Can you work these out from the model? Positions are in its coordinate system, mm. A direction names the side the tool comes from. Give positions to 0.01 mm unless a question says otherwise; leave off trailing zeros. Loops run counter-clockwise (first coordinate to the right, second up) from the corner with the lowest first, then second, coordinate; pieces in that order, holes last. Notation, with made-up numbers: (37.25, 70.5) -> (64.25, 70.5) arc R8 cw to (64.25, 83.5) -> close; hole circle Ø1 at (25.25, 35). An arc over 180 degrees is marked (long way). Return JSON: item names as keys, results as strings. Group by question number.
Q1. I need wall thicknesses on line 1 along X through (y, z) = (4.25, 10.5); line 2 along Y through (x, z) = (11, 0.75); line 3 along X through (y, z) = (13.5, 1.5) (3 decimals). Which ranges of each line are inside material? Lowest first, please. Write a range as [from, to].
Q2. Will these pins go through, and if not, where does the flat tip stop? pin 1 (0.8 mm diameter, centred on x = 0, z = 5.5, fed in from -Y); pin 2 (1 mm diameter, centred on y = 5, z = 2, fed in from -X); pin 3 (1.5 mm diameter, centred on x = 2.5, z = 5.5, fed in from +Y); pin 4 (1.5 mm diameter, centred on x = -4, y = 3, fed in from +Z).
Q3. Suppose I cut it at B-B, the plane z = 6. Please give me the cut outline in (x, y).
Q4. Suppose I cut it at C-C, the plane z = 1.5. Please give me the cut outline in (x, y).
Q5. Which directions (+Z, -Z, +X, -X, +Y, -Y) give clear straight access to the entire face, cutting with the end or side of a thin tool? Please do faces 1 (the cylindrical face through (3.101, 1.585, 5.916)), 2 (the flat face through (-2.8, 5, 6)), 3 (the cylindrical face through (2.16, 0.69, 5.92)).
Q6. Thinking about a two-plate mould opening in Y: for faces 4 (the flat face through (-1.5, 5, 6)), 5 (the cylindrical face through (2.14, 10.35, 9.34)), 6 (the cylindrical face through (-2.16, 10.35, 9.34)), 7 (the flat face through (10, 0, 6)), which applies, pulls with the +Y half, pulls with the -Y half, needs draft (parallel to the pull), parting line crosses it, or undercut?
Q7. Suppose I cut it at A-A, the plane y = 9.3. Please give me the cut outline in (x, z).
Q8. Suppose I cut it at D-D, the plane y = 7.5. Please give me the cut outline in (x, z).
```python
from build123d import *

# Parameters (mm, degrees)
EXTRUDE_1_DEPTH       = 12
HOLE_WIZARD_7_0_7_1_D = 7


with BuildPart() as part:
    # 草图1 → 拉伸-薄壁1 (new body)
    with BuildSketch(Plane.XY):
        with BuildLine():
            Line((-16.7, 0), (-3.8, 0))
            ThreePointArc((-3.8, 0), (-2.173654403, 0.673654403), (-1.5, 2.3))
            Line((-1.5, 2.3), (-1.5, 13))
            ThreePointArc((-1.5, 13), (-1.207106781, 13.707106781), (-0.5, 14))
            Line((-0.5, 14), (0.5, 14))
            ThreePointArc((0.5, 14), (1.207106781, 13.707106781), (1.5, 13))
            Line((1.5, 13), (1.5, 2.3))
            ThreePointArc((1.5, 2.3), (2.173654403, 0.673654403), (3.8, 0))
            Line((3.8, 0), (16.7, 0))
            Line((16.7, 0), (16.7, 1.3))
            Line((16.7, 1.3), (3.8, 1.3))
            ThreePointArc((3.8, 1.3), (3.092893219, 1.592893219), (2.8, 2.3))
            Line((2.8, 2.3), (2.8, 13))
            ThreePointArc((2.8, 13), (2.126345597, 14.626345597), (0.5, 15.3))
            Line((0.5, 15.3), (-0.5, 15.3))
            ThreePointArc((-0.5, 15.3), (-2.126345597, 14.626345597), (-2.8, 13))
            Line((-2.8, 13), (-2.8, 2.3))
            ThreePointArc((-2.8, 2.3), (-3.092893219, 1.592893219), (-3.8, 1.3))
            Line((-3.8, 1.3), (-16.7, 1.3))
            Line((-16.7, 1.3), (-16.7, 0))
        make_face()
    extrude(amount=EXTRUDE_1_DEPTH)

    # Ø7.0 (7) 直径孔1 (through all)
    with Locations(Plane(origin=(2.8, 0, 0), x_dir=(0, 0, -1), z_dir=(1, 0, 0))):
        with Locations((-6, 9.3)):
            Hole(HOLE_WIZARD_7_0_7_1_D / 2)


solid = part.part
```
Ans:
{
 "1": {"line 1": "x = [-2.8, -1.5], [1.5, 2.8]", "line 2": "y = [0, 1.3]", "line 3": "x = [-2.745, -1.366], [1.366, 2.745]"},
 "2": {"pin 1": "stops at y = 14", "pin 2": "stops at x = -2.8", "pin 3": "stops at y = 14.93", "pin 4": "passes through"},
 "3": {"outline": "(-16.7, 0) -> (-3.8, 0) arc R2.3 ccw to (-1.5, 2.3) -> (-1.5, 5.8) -> (-2.8, 5.8) -> (-2.8, 2.3) arc R1 cw to (-3.8, 1.3) -> (-16.7, 1.3) -> close; (-2.8, 12.8) -> (-1.5, 12.8) -> (-1.5, 13) arc R1 cw to (-0.5, 14) -> (0.5, 14) arc R1 cw to (1.5, 13) -> (1.5, 12.8) -> (2.8, 12.8) -> (2.8, 13) arc R2.3 ccw to (0.5, 15.3) -> (-0.5, 15.3) arc R2.3 ccw to (-2.8, 13) -> close; (1.5, 2.3) arc R2.3 ccw to (3.8, 0) -> (16.7, 0) -> (16.7, 1.3) -> (3.8, 1.3) arc R1 cw to (2.8, 2.3) -> (2.8, 5.8) -> (1.5, 5.8) -> close"},
 "4": {"outline": "(-16.7, 0) -> (-3.8, 0) arc R2.3 ccw to (-1.5, 2.3) -> (-1.5, 13) arc R1 cw to (-0.5, 14) -> (0.5, 14) arc R1 cw to (1.5, 13) -> (1.5, 2.3) arc R2.3 ccw to (3.8, 0) -> (16.7, 0) -> (16.7, 1.3) -> (3.8, 1.3) arc R1 cw to (2.8, 2.3) -> (2.8, 13) arc R2.3 ccw to (0.5, 15.3) -> (-0.5, 15.3) arc R2.3 ccw to (-2.8, 13) -> (-2.8, 2.3) arc R1 cw to (-3.8, 1.3) -> (-16.7, 1.3) -> close"},
 "5": {"face 1": "+Z, -Z, +X, +Y", "face 2": "+Z, -Z, -X, +Y", "face 3": "+Z, -Z, -Y"},
 "6": {"face 4": "needs draft", "face 5": "undercut", "face 6": "undercut", "face 7": "pulls with the -Y half"},
 "7": {"outline": "(-2.8, 0) -> (-1.5, 0) -> (-1.5, 2.5) -> (-2.8, 2.5) -> close; (-2.8, 9.5) -> (-1.5, 9.5) -> (-1.5, 12) -> (-2.8, 12) -> close; (1.5, 0) -> (2.8, 0) -> (2.8, 2.5) -> (1.5, 2.5) -> close; (1.5, 9.5) -> (2.8, 9.5) -> (2.8, 12) -> (1.5, 12) -> close"},
 "8": {"outline": "(-2.8, 0) -> (-1.5, 0) -> (-1.5, 3) -> (-2.8, 3) -> close; (-2.8, 9) -> (-1.5, 9) -> (-1.5, 12) -> (-2.8, 12) -> close; (1.5, 0) -> (2.8, 0) -> (2.8, 3) -> (1.5, 3) -> close; (1.5, 9) -> (2.8, 9) -> (2.8, 12) -> (1.5, 12) -> close"}
}
